```python
from build123d import *

# Parameters (mm, degrees)
F0_W     = 76.282457
F0_H     = 75.917773
F1_DEPTH = 50.45855
F2_R     = 15.096722
F3_DEPTH = 31.567339


with BuildPart() as f1:
    # F0 (on Front) → F1 (new body)
    with BuildSketch(Plane.XZ):
        with Locations((-38.141228, -37.958886)):
            Rectangle(F0_W, F0_H)
    extrude(amount=F1_DEPTH)

    # F2 (on face) → F3 (join)
    with BuildSketch(Plane.XY):
        with Locations((-31.907231, -26.368879)):
            Circle(F2_R)
    extrude(amount=F3_DEPTH)


solid = f1.part
```
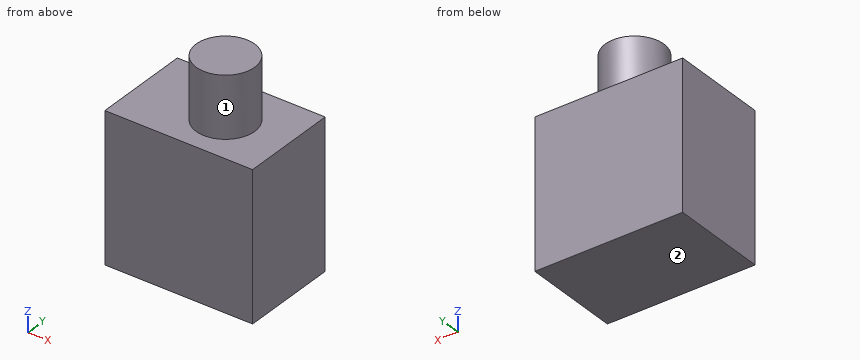
For this review, take the finished solid that the model builds, in its own axes (mm). Face numbers are marked on the shaded views. A direction names the side the tool comes from. Coordinates: 2 decimals unless noted, no trailing zeros. Loops run counter-clockwise (first coordinate to the right, second up) from the corner with the lowest first, then second, coordinate; pieces in that order, holes last. Notation, with made-up numbers: (3, -19.75) -> (15, -19.75) arc R19 cw to (15, -8.75) -> close; hole circle Ø9 at (88, 79.5). An arc over 180 degrees is marked (long way). Return JSON: item names as keys, results as strings. Group by question number.
(1) Consider section D-D, the plane x = -66. Give the boundary of the cut face in (y, z), plus the area to 3 significant figures.
(2) Consider section B-B, the plane x = -24. Give the boundary of the cut face in (y, z).
(3) Consider section C-C, the plane z = 22.5. Give the boundary of the cut face in (x, y), plus the area to 3 significant figures.
(4) For pin 1 Ø1 at (x, y) = (-64, -37.5) entering from +Z, flat-tipped, find the tip position at first contact; note if it passes through.
(5) To check wall thickness, follow L1, parallel to Z at x = -65, y = -5; L2, parallel to X at y = -26, z = 3.5; L3, parallel to X at y = -33, z = 9.5. State the ranges of each line that lie inside material, in increasing order.
(6) Tool access review of the marked faces 1 and 2: name each direction out of +Z, -Z, +X, -X, +Y, -Y from which nothing blocks a thin tool from reaching the whole face with its end or side.
(7) Consider section A-A, the plane y = -24.5. Give the boundary of the cut face in (x, z).
Results below:
{
 "1": {"outline": "(-50.46, -75.92) -> (0, -75.92) -> (0, 0) -> (-50.46, 0) -> close", "area": "3,830 mm2"},
 "2": {"outline": "(-50.46, -75.92) -> (0, -75.92) -> (0, 0) -> (-13.51, 0) -> (-13.51, 31.57) -> (-39.23, 31.57) -> (-39.23, 0) -> (-50.46, 0) -> close"},
 "3": {"outline": "circle Ø30.19 at (-31.91, -26.37)", "area": "716 mm2"},
 "4": {"pin 1": "stops at z = 0"},
 "5": {"L1": "z = -75.92 to 0", "L2": "x = -47 to -16.82", "L3": "x = -45.47 to -18.34"},
 "6": {"face 1": "+Z", "face 2": "-Z, +X, -X, +Y, -Y"},
 "7": {"outline": "(-76.28, -75.92) -> (0, -75.92) -> (0, 0) -> (-16.93, 0) -> (-16.93, 31.57) -> (-46.89, 31.57) -> (-46.89, 0) -> (-76.28, 0) -> close"}
}
